Input: part model. Units: mm. Frame: model coordinates. Face numbers are marked on the shaded views. A direction names the side the tool comes from. Round coordinates to 2 decimals unless told otherwise and drop trailing zeros. Order: outer loops, then holes, each group sorted by start corner. A loop starts at its lowest first (then second) coordinate and runs counter-clockwise, first axis right, second up.
Item 1: First-contact query: pin 1 (4 mm diameter, centred on x = -5, z = -86, fed in from -Y). Flat tip, straight axial feed; report the tip coordinate or a pass-through.
Item 2: Cut plane A-A on x = -5. Output: boundary loops of the cut face in (y, z) (3 decimals).
Item 3: Cut plane B-B on z = -53. Output: boundary loops of the cut face in (x, y), then the cut area to 3 significant figures.
Item 4: Reachability of the marked faces 1 and 2 from +Z, -Z, +X, -X, +Y, -Y: full face, straight path, thin tool, end or side. Return the list, or none.
Item 5: Line query: L1, parallel to Z at x = -5, y = 10.25; L2, parallel to X at y = 9.5, z = -86; L3, parallel to X at y = 12.5, z = -43. Output: solid intervals per line, ascending.
Item 6: Cut plane C-C on x = -34. Output: boundary loops of the cut face in (y, z).
Item 7: Mould query, pull axis X, two halves, no side actions, for the marked faces 3, 4, 5 and 6. Classes: released by +X, released by -X, zero draft, split by the parting line, or undercut.
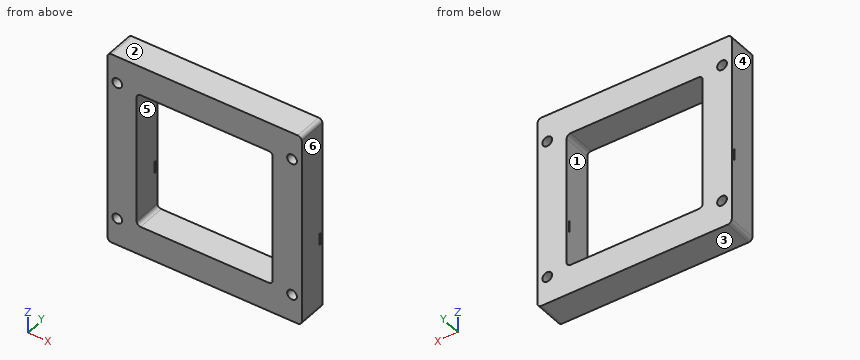
Autodesk Inventor part; units mm, degrees
ref_plane "YZ Plane" through (0, 0, 0) normal (1, 0, 0) x (0, 1, 0)
ref_plane "XZ Plane" through (0, 0, 0) normal (0, 1, 0) x (-1, 0, 0)
ref_plane "XY Plane" through (0, 0, 0) normal (0, 0, 1) x (1, 0, 0)
sketch "Szkic1" plane through (0, 0, 0) normal (0, 1, 0) x (-1, 0, 0)
  line L0 (0, 0) -> (100, 0)
  line L1 (100, 0) -> (100, -100)
  line L2 (100, -100) -> (0, -100)
  line L3 (0, -100) -> (0, 0)
  dimension "d0" = 100
  dimension "d1" = 100
sketch "Szkic2" plane through (0, 0, 0) normal (0, 1, 0) x (-1, 0, 0)
  line L0 (15, -15) -> (85, -15)
  line L1 (85, -15) -> (85, -85)
  line L2 (85, -85) -> (15, -85)
  line L3 (15, -85) -> (15, -15)
  point P0 (0, 0)
  dimension "d2" = 70
  dimension "d3" = 70
  dimension "d4" = 15
  dimension "d5" = 15
extrude "Wyciągnięcie proste1" add sketch "Szkic1" along normal blind 15
extrude "Wyciągnięcie proste2" cut sketch "Szkic2" along normal blind 15
fillet "Zaokrąglenie1" radius 2 8 edges at (-85, 7.5, -85) (-15, 7.5, -85) (-15, 7.5, -15) (-85, 7.5, -15) (-100, 7.5, 0) (-100, 7.5, -100) (0, 7.5, -100) (0, 7.5, 0)
sketch "Szkic3" plane through (0, 15, 0) normal (0, 1, 0) x (1, 0, 0)
  line L0 (0, 2) -> (0, 98)
  line L1 (-2, 100) -> (-98, 100)
  line L2 (-98, 0) -> (-2, 0)
  line L3 (-100, 98) -> (-100, 2)
  point P0 (0, 0)
  point P1 (-5, 86)
  point P2 (-5, 14)
  point P3 (-95, 86)
  point P4 (-95, 14)
  dimension "d11" = 5
  dimension "d12" = 14
  dimension "d13" = 14
  dimension "d14" = 14
  dimension "d15" = 5
  dimension "d16" = 5
  dimension "d17" = 5
  dimension "d18" = 14
hole "Otwór1" at (-5, 15, -86) at (-5, 15, -14) at (-95, 15, -86) at (-95, 15, -14) direction (0, -1, 0) diameter 5 depth 15
sketch "Szkic4" plane through (0, 15, 0) normal (0, 1, 0) x (1, 0, 0)
  point P0 (0, 0)
sketch "Szkic5" plane through (0, 0, -2) normal (1, 0, 0) x (0, 0, -1)
  line L0 (57.525, 13.5) -> (63.525, 13.5)
  line L1 (63.525, 13.5) -> (63.525, 13)
  line L2 (63.525, 13) -> (57.525, 13)
  line L3 (57.525, 13) -> (57.525, 13.5)
  line L4 (0, 15) -> (96, 15)
  line L5 (98, 0) -> (98, 15)
  point P0 (-2, 0)
  point P1 (63.525, 13.25)
  dimension "d26" = 6
  dimension "d27" = 0.5
  dimension "d28" = 1.5
  dimension "d29" = 34.475
extrude "Wyciągnięcie proste3" cut sketch "Szkic5" against normal through all
equation "\"d1\" = d0"
properties part number "podstawka_prowadzaca"
From the geometry:
1. pin 1: passes through
2. outline: (0, -100) - (15, -100) - (15, -88.5) - (0, -88.5) - close; (0, -83.5) - (15, -83.5) - (15, -16.5) - (0, -16.5) - close; (0, -11.5) - (15, -11.5) - (15, 0) - (0, 0) - close; hole (13, -65.525) - (13.5, -65.525) - (13.5, -59.525) - (13, -59.525) - close
3. outline: (-100, 0) - (-85, 0) - (-85, 15) - (-100, 15) - close; (-15, 0) - (0, 0) - (0, 15) - (-15, 15) - close
3. area: 450 mm2
4. face 1: +Y, -Y
4. face 2: +Z, +X, -X, +Y, -Y
5. L1: z = -100 to -88.5, -83.5 to -16.5, -11.5 to 0
5. L2: x = -100 to -97.5, -92.5 to -7.5, -2.5 to 0
5. L3: x = -100 to -85, -15 to 0
6. outline: (0, -100) - (15, -100) - (15, -85) - (0, -85) - close; (0, -15) - (15, -15) - (15, 0) - (0, 0) - close
7. face 3: zero draft
7. face 4: released by -X
7. face 5: undercut
7. face 6: released by +X
